Check sheet for the modelled part. Datum: model origin and axes. Units: mm. Coordinates: 2 decimals unless noted, no trailing zeros. Write each loop counter-clockwise with the first axis right and the second up, starting at its lowest first coordinate (ties: lowest second). Pieces come first, ordered by that corner, then holes. Notation, with made-up numbers: M 62.5,11.25 L 108.5,11.25 A16 ccw 108.5,16.25 Z; hole C 3.5,87.5 d5. An arc over 180 degrees is marked long. Answer as CSV lines item,"result".
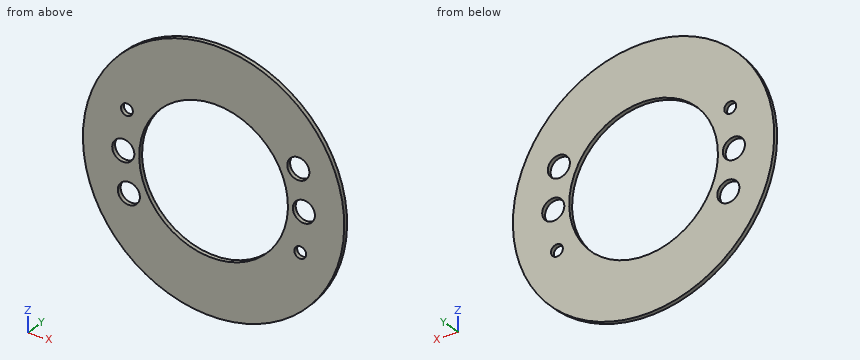
from build123d import *

# Parameters (mm, degrees)
SKETCH1_R           = 78.105
SKETCH1_R_2         = 44.45
BOSS_EXTRUDE1_DEPTH = 2.54
SKETCH2_R           = 6.604
SKETCH2_R_2         = 3.556
CUT_EXTRUDE1_DEPTH  = 2.54


with BuildPart() as part:
    # Sketch1 → Boss-Extrude1 (new body)
    with BuildSketch(Plane(origin=(0, 0, 0), x_dir=(1, 0, 0), z_dir=(0, 1, 0))):
        with Locations(Location((0, 0, 0), (0, 0, 270))):
            Circle(SKETCH1_R)
        with Locations(Location((0, 0, 0), (0, 0, 270))):
            Circle(SKETCH1_R_2, mode=Mode.SUBTRACT)
    extrude(amount=BOSS_EXTRUDE1_DEPTH)

    # Sketch2 → Cut-Extrude1 (cut)
    with BuildSketch(Plane(origin=(0, 2.54, 0), x_dir=(1, 0, 0), z_dir=(0, 1, 0))):
        with Locations(Location((-53.975, 0, 0), (0, 0, 270))):
            Circle(SKETCH2_R)
        with Locations(Location((53.975, 0, 0), (0, 0, 270))):
            Circle(SKETCH2_R)
        with Locations(Location((-51.795490029, -24.152633658, 0), (0, 0, 270))):
            Circle(SKETCH2_R_2)
        with Locations(Location((51.795490029, 24.152633658, 0), (0, 0, 270))):
            Circle(SKETCH2_R_2)
        with Locations(Location((50.64447914, -23.615908466, 0), (0, 0, 270))):
            Circle(SKETCH2_R)
        with Locations(Location((-50.64447914, 23.615908466, 0), (0, 0, 270))):
            Circle(SKETCH2_R)
    extrude(amount=-CUT_EXTRUDE1_DEPTH, mode=Mode.SUBTRACT)


solid = part.part
1) Section check A-A, the plane x = 0. Record the boundary of the cut face in (y, z) (3 decimals), plus the area to 3 significant figures.
Answer key:
outline,"M 0,-78.105 L 2.54,-78.105 L 2.54,-44.45 L 0,-44.45 Z; M 0,44.45 L 2.54,44.45 L 2.54,78.105 L 0,78.105 Z"
area,"171 mm2"
2) Section check D-D, the plane x = -19. Record the boundary of the cut face in (y, z), plus the area to 3 significant figures.
Answer key:
outline,"M 0,-75.76 L 2.54,-75.76 L 2.54,-40.18 L 0,-40.18 Z; M 0,40.18 L 2.54,40.18 L 2.54,75.76 L 0,75.76 Z"
area,"181 mm2"
3) Section check C-C, the plane y = 2.05. Give the number of separate pieces and of enclosed holes in the cut face, plus the area to 3 significant figures.
Answer key:
separate pieces,"1"
enclosed holes,"7"
area,"12,300 mm2"
4) Section check B-B, the plane z = 0. Record the boundary of the cut face in (x, y) (3 decimals).
Answer key:
outline,"M -78.105,0 L -60.579,0 L -60.579,2.54 L -78.105,2.54 Z; M -47.371,0 L -44.45,0 L -44.45,2.54 L -47.371,2.54 Z; M 44.45,0 L 47.371,0 L 47.371,2.54 L 44.45,2.54 Z; M 60.579,0 L 78.105,0 L 78.105,2.54 L 60.579,2.54 Z"
5) Depth check by flat-ended pin: P1, Ø17, axis at x = 50.64, z = 23.62, coming from the -Y side. Enter the tip coordinate at first touch or a pass-through.
Answer key:
P1,"stops at y = 0"
6) Thickness scan on line 1 along X through (y, z) = (0.5, 0) (3 decimals); line 2 along X through (y, z) = (0.6, -21.5); line 3 along Z through (x, y) = (20, 1.35). Record the ranges inside material, lowest first.
Answer key:
line 1,"x = -78.105 to -60.579, -47.371 to -44.45, 44.45 to 47.371, 60.579 to 78.105"
line 2,"x = -75.09 to -56.9, -44.39 to -38.9, 38.9 to 49.43, 54.16 to 75.09"
line 3,"z = -75.5 to -39.7, 39.7 to 75.5"
